Could you check a few things on this model? Use its own coordinates, in mm. A direction names the side the tool comes from. Round coordinates to 2 decimals unless told otherwise and drop trailing zeros. Write each loop counter-clockwise with the first axis right and the second up, starting at its lowest first coordinate (ties: lowest second). Pieces come first, ordered by that corner, then holes. Notation, with made-up numbers: (-4.75, -26.5) -> (40.25, -26.5) arc R24 ccw to (40.25, 10.5) -> close; hole circle Ø9 at (-15.75, 42.5). An arc over 180 degrees is marked (long way). Answer in a Markdown table with one row per item.
from build123d import *

# Parameters (mm, degrees)
SKETCH6_W            = 10.1981
SKETCH6_H            = 4.28752
BOSS_EXTRUDE3_DEPTH  = 25.4
SKETCH8_R            = 5.09905
BOSS_EXTRUDE5_DEPTH  = 19.05
SKETCH11_W           = 65.69456
SKETCH11_H           = 25.654
BOSS_EXTRUDE10_DEPTH = 4.28752
SKETCH16_W           = 1.143
SKETCH16_H           = 5.08
SKETCH16_W_2         = 1.155076163
BOSS_EXTRUDE11_DEPTH = 38.0746
SKETCH17_W           = 26.52268
SKETCH17_H           = 5.08
BOSS_EXTRUDE12_DEPTH = 4.5212
FILLET2_R            = 2.54
FILLET3_R            = 2.54
FILLET4_R            = 2.54


with BuildPart() as part:
    # Sketch6 → Boss-Extrude3 (new body)
    with BuildSketch(Plane(origin=(0, 0, 0), x_dir=(1, 0, 0), z_dir=(0, 1, 0))):
        with Locations((-12.169797761, 9.77580804)):
            Rectangle(SKETCH6_W, SKETCH6_H)
    extrude(amount=BOSS_EXTRUDE3_DEPTH)

    # Sketch8 → Boss-Extrude5 (add)
    with BuildSketch(Plane.XY.offset(-11.91956804)):
        with Locations((-12.169797761, 5.098542)):
            Circle(SKETCH8_R)
    extrude(amount=-BOSS_EXTRUDE5_DEPTH)

    # Sketch11 → Boss-Extrude10 (add)
    with BuildSketch(Plane(origin=(0, 25.4, 0), x_dir=(1, 0, 0), z_dir=(0, 1, 0))):
        with Locations((-12.150747761, 20.45904804)):
            Rectangle(SKETCH11_W, SKETCH11_H)
    extrude(amount=BOSS_EXTRUDE10_DEPTH)

    # Sketch16 → Boss-Extrude11 (add)
    with BuildSketch(Plane(origin=(0, 29.68752, 0), x_dir=(1, 0, 0), z_dir=(0, 1, 0))):
        with Locations((-44.426527761, 20.45904804)):
            Rectangle(SKETCH16_W, SKETCH16_H)
        with Locations((20.118994158, 20.45904804)):
            Rectangle(SKETCH16_W_2, SKETCH16_H)
    extrude(amount=BOSS_EXTRUDE11_DEPTH)

    # Sketch17 → Boss-Extrude12 (add)
    with BuildSketch(Plane(origin=(0, 67.76212, 0), x_dir=(1, 0, 0), z_dir=(0, 1, 0))):
        with Locations((-31.736687761, 20.45904804)):
            Rectangle(SKETCH17_W, SKETCH17_H)
        with Locations((7.435192239, 20.45904804)):
            Rectangle(SKETCH17_W, SKETCH17_H)
    extrude(amount=BOSS_EXTRUDE12_DEPTH)

    # Fillet2
    fillet2_edges = [part.edges().sort_by_distance(p)[0] for p in [
        (-12.169797761, 25.4, -11.91956804),
    ]]
    fillet(fillet2_edges, radius=FILLET2_R)

    # Fillet3
    fillet3_edges = [part.edges().sort_by_distance(p)[0] for p in [
        (-17.268847761, 25.4, -11.04580804),
    ]]
    fillet(fillet3_edges, radius=FILLET3_R)

    # Fillet4
    fillet4_edges = [part.edges().sort_by_distance(p)[0] for p in [
        (-7.070747761, 25.4, -11.04580804),
    ]]
    fillet(fillet4_edges, radius=FILLET4_R)


solid = part.part
1) Imagine slicing it at B-B, the plane x = 1. Please give me the cut outline in (y, z), plus the area to 3 significant figures.
Findings:
| item | result |
|---|---|
| outline | (25.4, -33.29) -> (29.69, -33.29) -> (29.69, -7.63) -> (25.4, -7.63) -> close; (67.76, -23) -> (72.28, -23) -> (72.28, -17.92) -> (67.76, -17.92) -> close |
| area | 133 mm^2 |
2) Imagine slicing it at A-A, the plane y = 43. Please give me the cut outline in (x, z).
Findings:
| item | result |
|---|---|
| outline | (-45, -23) -> (-43.86, -23) -> (-43.86, -17.92) -> (-45, -17.92) -> close; (19.54, -23) -> (20.7, -23) -> (20.7, -17.92) -> (19.54, -17.92) -> close |
3) Please list where these lines run through material, in increasing order: line 1 (Y direction, x = -5, z = -18); line 2 (Y direction, x = 1, z = -29); line 3 (Z direction, x = -33, y = 68.5).
Findings:
| item | result |
|---|---|
| line 1 | y = 25.4 to 29.69, 67.76 to 72.28 |
| line 2 | y = 25.4 to 29.69 |
| line 3 | z = -23 to -17.92 |
4) Imagine slicing it at D-D, the plane x = -16. Please give me the cut outline in (y, z).
Findings:
| item | result |
|---|---|
| outline | (0, -11.92) -> (1.73, -11.92) -> (1.73, -30.97) -> (8.46, -30.97) -> (8.46, -11.92) -> (22.86, -11.92) arc R2.54 cw to (25.4, -14.46) -> (25.4, -33.29) -> (29.69, -33.29) -> (29.69, -7.63) -> (0, -7.63) -> close |
5) Thinking about a two-plate mould opening in X: for faces 6 (the face through (7, 67.762, -20)), 7 (the face through (-13, 25.4, -21)), 8 (the face through (-7.071, 11, -10)), which applies, +X half, -X half, draft (parallel to the pull), parting line (faces both ways), or undercut?
Findings:
| item | result |
|---|---|
| face 6 | undercut |
| face 7 | draft |
| face 8 | +X half |
6) For faces 1 (the face through (-35, 68, -17.919)), 2 (the face through (10, 68, -22.999)), 3 (the face through (-17.269, 11, -10)), 4 (the face through (-12.063, 24.636, -12.644)), 5 (the face through (-16, 1, -11.92)), which set-ups out of +Z, -Z, +X, -X, +Y, -Y let a thin tool reach every point of the face, with its end or its side?
Findings:
| item | result |
|---|---|
| face 1 | +Z, +X, -X, +Y |
| face 2 | -Z, +X, -X, +Y |
| face 3 | +Z, -Z, -X, -Y |
| face 4 | -Z, +X, -X |
| face 5 | -Z, -X, -Y |
7) Imagine slicing it at C-C, the plane z = -29.5. Please give me the cut outline in (x, y), plus the area to 3 significant figures.
Findings:
| item | result |
|---|---|
| outline | (-45, 25.4) -> (20.7, 25.4) -> (20.7, 29.69) -> (-45, 29.69) -> close; circle Ø10.2 at (-12.17, 5.1) |
| area | 363 mm^2 |
8) For pin 1 (11 mm diameter, centred on x = -12, y = 5.5, fed in from -Z); pin 2 (4 mm diameter, centred on x = -33, z = -21.5, fed in from -Y); pin 3 (1.5 mm diameter, centred on y = 10, z = -16, fed in from -X), each with a flat end and sliding along its axis, tell me the tip position at first contact or that it passes through.
Findings:
| item | result |
|---|---|
| pin 1 | stops at z = -30.97 |
| pin 2 | stops at y = 25.4 |
| pin 3 | stops at x = -15.13 |
